Work out the finished part from the listing and answer in its coordinate system (mm). Coordinates: 2 decimals unless noted, no trailing zeros. Loops run counter-clockwise (first coordinate to the right, second up) from the corner with the lowest first, then second, coordinate; pieces in that order, holes last. Notation, with made-up numbers: (-1, -32.5) -> (18, -32.5) arc R12 ccw to (18, -23.5) -> close; hole circle Ø7 at (39, 8). An arc over 180 degrees is marked (long way). Use a Markdown table: item, result.
from build123d import *

# Parameters (mm, degrees)
EXTRUDE_1_DEPTH     = 1.4
SKETCH_3_R          = 1.5
CUT_EXTRUDE_1_DEPTH = 3.8
FILLET_1_R          = 0.2


with BuildPart() as part:
    # 草图1 → 凸台-拉伸1 (new body, symmetric)
    with BuildSketch(Plane(origin=(0, 0, 0), x_dir=(1, 0, 0), z_dir=(0, 1, 0))):
        Polygon((3.117691454, 0), (1.558845727, 2.7), (-1.558845727, 2.7), (-3.117691454, 0), (-1.558845727, -2.7), (1.558845727, -2.7), align=None)
    extrude(amount=EXTRUDE_1_DEPTH, both=True)

    # 草图2 → 切除-旋转1 (revolve, cut)
    with BuildSketch(Plane.XY):
        Polygon((-3.117691454, 1.1), (-2.5, 1.4), (-3.117691454, 1.4), align=None)
    cut_revolve_1 = revolve(axis=Axis((0, 0, 0), (0, 1, 0)), mode=Mode.SUBTRACT)

    # 镜向3: 切除-旋转1 across plane
    add(cut_revolve_1.mirror(Plane.ZX), mode=Mode.SUBTRACT)

    # 草图3 → 切除-拉伸1 (cut, through all)
    with BuildSketch(Plane(origin=(0, 1.4, 0), x_dir=(1, 0, 0), z_dir=(0, 1, 0))):
        Circle(SKETCH_3_R)
    extrude(amount=-CUT_EXTRUDE_1_DEPTH, mode=Mode.SUBTRACT)

    # 草图4 → 旋转1 (revolve)
    with BuildSketch(Plane(origin=(0, 0, 0), x_dir=(0, 0, -1), z_dir=(1, 0, 0))):
        with BuildLine():
            Line((-2.5, 1.4), (-2.5, 1.6))
            ThreePointArc((-2.5, 1.6), (-2.353553391, 1.953553391), (-2, 2.1))
            Line((-2, 2.1), (-1.5, 2.1))
            Line((-1.5, 2.1), (-1.5, 1.4))
            Line((-1.5, 1.4), (-2.5, 1.4))
        make_face()
    revolve(axis=Axis((0, 1.4, 0), (0, -1, 0)))

    # 圆角1
    fillet_1_edges = [part.edges().sort_by_distance(p)[0] for p in [
        (-1.767766953, 1.4, 1.767766953),
        (0, 2.1, -1.5),
    ]]
    fillet(fillet_1_edges, radius=FILLET_1_R)


solid = part.part
Q1. Section A-A on y = 1.7 is taken. Determine the outline of the cut face in (x, z), and give its area (3 significant figures).
Solved:
| item | result |
|---|---|
| outline | circle Ø4.98 at (0, 0); hole circle Ø3 at (0, 0) |
| area | 12.4 mm² |
Q2. Consider line 1 (Z direction, x = 0, y = -0.1); line 2 (X direction, y = 1.75, z = 0); line 3 (Z direction, x = 0.5, y = 1.7). Determine where each line is inside the solid, lowest interval first. Write a range as [from, to].
Solved:
| item | result |
|---|---|
| line 1 | [-2.7, -1.5], [1.5, 2.7] |
| line 2 | [-2.48, -1.5], [1.5, 2.48] |
| line 3 | [-2.44, -1.41], [1.41, 2.44] |
Q3. Given pin 1 Ø1.5 at (y, z) = (1.5, 1) entering from +X; pin 2 Ø2.5 at (x, z) = (0, 0) entering from +Y, each flat-ended and moving along its own axis, determine where each tip first touches the part or whether it passes through.
Solved:
| item | result |
|---|---|
| pin 1 | x = 2.93 |
| pin 2 | through |
